For this review, take the finished solid that the model builds, in its own axes (mm). A direction names the side the tool comes from. Give positions to 0.01 mm unless a question says otherwise; leave off trailing zeros. Order: outer loops, then holes, each group sorted by start corner. A loop starts at its lowest first (then second) coordinate and runs counter-clockwise, first axis right, second up. Notation, with made-up numbers: (-31.75, 69) -> (6.25, 69) arc R14 cw to (6.25, 93) -> close; hole circle Ø8 at (74, -13.75). An arc over 180 degrees is marked (long way). One line per item, written item: value. Start each with the question number.
from build123d import *

# Parameters (mm, degrees)
F0_R      = 5.5
F1_DEPTH  = 1
F2_R      = 4.5
F3_DEPTH  = 1.5
F4_R      = 4
F5_DEPTH  = 5
F6_R      = 4
F7_R      = 4
F8_DEPTH  = 13.3
F9_W      = 0.5
F9_H      = 0.5
F10_DEPTH = 15.5
F11_W     = 0.5
F11_H     = 0.5
F12_DEPTH = 1.5


with BuildPart() as f1:
    # F0 (on Top) → F1 (new body)
    with BuildSketch(Plane.XY):
        Circle(F0_R)
    extrude(amount=F1_DEPTH)

    # F2 (on face) → F3 (join)
    with BuildSketch(Plane.XY.offset(1)):
        Circle(F2_R)
    extrude(amount=F3_DEPTH)

    # F4 (on face) → F5 (join)
    with BuildSketch(Plane.XY.offset(2.5)):
        Circle(F4_R)
    extrude(amount=F5_DEPTH)

    # F6
    f6_edges = [f1.edges().sort_by_distance(p)[0] for p in [
        (-4, 0, 7.5),
    ]]
    fillet(f6_edges, radius=F6_R)

    # F7 (on face) → F8 (join)
    with BuildSketch(Plane(origin=(0, 0, 0), x_dir=(1, 0, 0), z_dir=(0, 0, -1))):
        Circle(F7_R)
    extrude(amount=F8_DEPTH)

    # F9 (on face) → F10 (join)
    with BuildSketch(Plane(origin=(0, 0, -13.3), x_dir=(1, 0, 0), z_dir=(0, 0, -1))):
        with Locations((-1.27, 0)):
            Rectangle(F9_W, F9_H)
        with Locations((1.27, 0)):
            Rectangle(F9_W, F9_H)
    extrude(amount=F10_DEPTH)

    # F11 (on face) → F12 (join)
    with BuildSketch(Plane(origin=(0, 0, -28.8), x_dir=(1, 0, 0), z_dir=(0, 0, -1))):
        with Locations((-1.27, 0)):
            Rectangle(F11_W, F11_H)
    extrude(amount=F12_DEPTH)


solid = f1.part
Q1. Take a section at B-B (x = 0). State the section outline as (y, z) points, and give its area (3 significant figures).
Q2. Take a section at D-D (z = -1.5). State the section outline as (x, y) points, and give its area (3 significant figures).
Q3. For faces 1 (the cylindrical face through (-0.867, -3.905, 2.993)), 2 (the cylindrical face through (-1.19, -5.37, 0.49)), 3 (the cylindrical face through (-0.867, 3.905, -6.557)), list the 3-axis set-ups (+Z, -Z, +X, -X, +Y, -Y) from which the entire face can be reached by the end or side of a thin tool; tool diameter is ignored.
Q4. For pin 1 Ø4 at (y, z) = (-3, -10) entering from +X; pin 2 Ø6 at (x, y) = (2, 4) entering from +Z; pin 3 Ø0.6 at (x, z) = (-1.5, -18.5) entering from +Y, all flat-tipped, find the tip position at first contact; note any pin that passes through.
Q5. Take a section at C-C (y = -3.5). State the section outline as (x, z) points, and give its area (3 significant figures).
Q6. For line 1 along Z through (x, y) = (1.75, -4.5); line 2 along Y through (x, z) = (0, -3.5); line 3 along X through (y, z) = (0.25, -12), list the stretches that pass through material, from the lowest coordinate up.
Q7. Take a section at A-A (z = -23). State the section outline as (x, y) points.
Answers below:
1. outline: (-5.5, 0) -> (-4, 0) -> (-4, -13.3) -> (4, -13.3) -> (4, 0) -> (5.5, 0) -> (5.5, 1) -> (4.5, 1) -> (4.5, 2.5) -> (4, 2.5) -> (4, 3.5) arc R4 ccw to (-4, 3.5) -> (-4, 2.5) -> (-4.5, 2.5) -> (-4.5, 1) -> (-5.5, 1) -> close
1. area: 164 mm²
2. outline: circle Ø8 at (0, 0)
2. area: 50.3 mm²
3. face 1: +Z
3. face 2: +Z, -Z
3. face 3: -Z
4. pin 1: stops at x = 3.87
4. pin 2: stops at z = 7.22
4. pin 3: stops at y = 0.25
5. outline: (-4.24, 0) -> (-1.94, 0) -> (-1.94, -13.3) -> (1.94, -13.3) -> (1.94, 0) -> (4.24, 0) -> (4.24, 1) -> (2.83, 1) -> (2.83, 2.5) -> (1.94, 2.5) -> (1.94, 3.5) arc R1.94 ccw to (-1.94, 3.5) -> (-1.94, 2.5) -> (-2.83, 2.5) -> (-2.83, 1) -> (-4.24, 1) -> close
5. area: 78.2 mm²
6. line 1: z = 0 to 1
6. line 2: y = -4 to 4
6. line 3: x = -3.99 to 3.99
7. outline: (-1.52, -0.25) -> (-1.02, -0.25) -> (-1.02, 0.25) -> (-1.52, 0.25) -> close; (1.02, -0.25) -> (1.52, -0.25) -> (1.52, 0.25) -> (1.02, 0.25) -> close
